Geometry: final body of the model. Coordinates: model frame, mm. Face numbers are marked on the shaded views. A direction names the side the tool comes from. Round coordinates to 2 decimals unless told otherwise and drop trailing zeros. Loops run counter-clockwise (first coordinate to the right, second up) from the corner with the lowest first, then second, coordinate; pieces in that order, holes last. Notation, with made-up numbers: (77.25, 43.5) -> (83.25, 43.5) arc R25 cw to (83.25, 64.5) -> close; hole circle Ø6 at (56, 27.25). An arc over 180 degrees is marked (long way). Answer in a Markdown table with one row per item.
Autodesk Inventor part; units mm, degrees
ref_plane "YZ Plane" through (0, 0, 0) normal (1, 0, 0) x (0, 1, 0)
ref_plane "XZ Plane" through (0, 0, 0) normal (0, 1, 0) x (-1, 0, 0)
ref_plane "XY Plane" through (0, 0, 0) normal (0, 0, 1) x (1, 0, 0)
sketch "Sketch1" plane through (0, 0, 0) normal (0, 1, 0) x (-1, 0, 0)
  circle A0 centre (0, 0) radius 17.5
  dimension "d0" = 35
extrude "Extrusion1" add sketch "Sketch1" along normal mid plane 2.5
sketch "Sketch2" plane through (0, 1.25, 0) normal (0, 1, 0) x (1, 0, 0)
  circle A0 centre (0, 0) radius 10.25
  dimension "d3" = 20.5
extrude "Extrusion2" add sketch "Sketch2" along normal blind 1
sketch "Sketch3" plane through (0, -1.25, 0) normal (0, -1, 0) x (1, 0, 0)
  circle A0 centre (0, 0) radius 9.5
  dimension "d6" = 19
extrude "Extrusion3" add sketch "Sketch3" along normal blind 0.5
sketch "Sketch4" plane through (0, 1.25, 0) normal (0, 1, 0) x (1, 0, 0)
  circle A0 centre (0, 14.5) radius 1.5
  circle A1 centre (-13.7903, 4.4807) radius 1.5
  circle A2 centre (-8.5229, -11.7307) radius 1.5
  circle A3 centre (8.5229, -11.7307) radius 1.5
  circle A4 centre (13.7903, 4.4807) radius 1.5
  point P0 (0, 0)
  dimension "d9" = 3
  dimension "d10" = 14.5
  dimension "d13" = 360
extrude "Extrusion4" cut sketch "Sketch4" against normal through all
properties material "Iron, Cast"
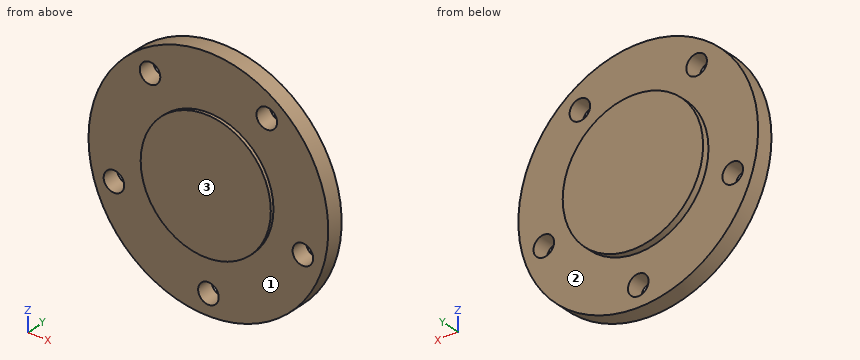
Item 1: Section query B-B, the plane z = -15. Output: boundary loops of the cut face in (x, y).
Ans:
| item | result |
|---|---|
| outline | (-9.01, -1.25) -> (-1.41, -1.25) -> (-1.41, 1.25) -> (-9.01, 1.25) -> close; (1.41, -1.25) -> (9.01, -1.25) -> (9.01, 1.25) -> (1.41, 1.25) -> close |
Item 2: Section query C-C, the plane z = 0. Output: boundary loops of the cut face in (x, y), and give its area (4 significant figures).
Ans:
| item | result |
|---|---|
| outline | (-17.5, -1.25) -> (-9.5, -1.25) -> (-9.5, -1.75) -> (9.5, -1.75) -> (9.5, -1.25) -> (17.5, -1.25) -> (17.5, 1.25) -> (10.25, 1.25) -> (10.25, 2.25) -> (-10.25, 2.25) -> (-10.25, 1.25) -> (-17.5, 1.25) -> close |
| area | 117.5 mm2 |
Item 3: Set-up query: the marked faces 1, 2 and 3. Return all of +Z, -Z, +X, -X, +Y, -Y with unobstructed straight access to the full face (end or side cutting, diameter ignored); none if empty.
Ans:
| item | result |
|---|---|
| face 1 | -Y |
| face 2 | +Y |
| face 3 | +Z, -Z, +X, -X, -Y |
Item 4: First-contact query: P1, Ø1.5, axis at x = -11, z = -10, coming from the +Y side; P2, Ø1.8, axis at x = -13.79, z = -4.48, coming from the +Y side; P3, Ø2, axis at y = 1.5, z = 10, coming from the -X side; P4, Ø1.5, axis at y = 1, z = 3.5, coming from the -X side. Flat tips, straight axial feed; report the tip coordinate or a pass-through.
Ans:
| item | result |
|---|---|
| P1 | y = 1.25 |
| P2 | through |
| P3 | x = -14.99 |
| P4 | x = -17.28 |
Item 5: Section query A-A, the plane x = 0. Output: boundary loops of the cut face in (y, z), and give its area (3 significant figures).
Ans:
| item | result |
|---|---|
| outline | (-1.75, -9.5) -> (-1.25, -9.5) -> (-1.25, -13) -> (1.25, -13) -> (1.25, -10.25) -> (2.25, -10.25) -> (2.25, 10.25) -> (1.25, 10.25) -> (1.25, 17.5) -> (-1.25, 17.5) -> (-1.25, 9.5) -> (-1.75, 9.5) -> close; (-1.25, -17.5) -> (1.25, -17.5) -> (1.25, -16) -> (-1.25, -16) -> close |
| area | 110 mm2 |
Item 6: Ray query, L1, parallel to Z at x = 0, y = 0.45; L2, parallel to Z at x = -8.5, y = -0.7; L3, parallel to Y at x = 9, z = 13.5. Return the intervals inside material, ascending.
Ans:
| item | result |
|---|---|
| L1 | -17.5 to -16, -13 to 17.5 |
| L2 | -15.3 to 10.23, 13.23 to 15.3 |
| L3 | -1.25 to 1.25 |
Item 7: Section query D-D, the plane y = -0.4. Output: boundary loops of the cut face in (x, z).
Ans:
| item | result |
|---|---|
| outline | circle Ø35 at (0, 0); hole circle Ø3 at (-13.79, -4.48); hole circle Ø3 at (-8.52, 11.73); hole circle Ø3 at (0, -14.5); hole circle Ø3 at (8.52, 11.73); hole circle Ø3 at (13.79, -4.48) |
